Part model, mm, in its own coordinate system. A direction names the side the tool comes from. Round coordinates to 2 decimals unless told otherwise and drop trailing zeros. Loops run counter-clockwise (first coordinate to the right, second up) from the corner with the lowest first, then second, coordinate; pieces in that order, holes last. Notation, with made-up numbers: (5.25, 80) -> (14.25, 80) arc R21 cw to (14.25, 103) -> close; hole circle Ø7 at (69.25, 60.5). An arc over 180 degrees is marked (long way). Answer as a JSON object with one key per item and string values. Group by question number.
from build123d import *

# Parameters (mm, degrees)
CUT_EXTRUDE1_DEPTH      = 127.059509756
CUT_EXTRUDE1_DEPTH_BACK = 127.059509756
SKETCH3_OUTSIDE_W       = 84.264
SKETCH3_OUTSIDE_H       = 84.264
SKETCH3_OUTSIDE_R       = 19
CHAMFER1_SIZE           = 1
CUT_EXTRUDE2_DEPTH      = 148.885090526
CUT_EXTRUDE2_DEPTH_BACK = 148.885090526
SKETCH6_R               = 5
CHAMFER3_SIZE           = 2


with BuildPart() as part:
    # Sketch2 → Revolve1 (revolve)
    with BuildSketch(Plane.XY, mode=Mode.PRIVATE) as revolve1_sk:
        Polygon((0, 0), (145, 0), (145, 15), (39, 15), (39, 25), (24, 25), (24, 15.2), (0, 15.2), align=None)
    revolve(revolve1_sk.sketch.rotate(Axis((0, 0, 0), (1, 0, 0)), 90), axis=Axis((0, 0, 0), (1, 0, 0)))

    # Sketch3 outside → Cut-Extrude1 (cut, two sides: drawn at the far end of the back side and taken through both)
    with BuildSketch(Plane.ZY.offset(-24).offset(-CUT_EXTRUDE1_DEPTH_BACK)):
        Rectangle(SKETCH3_OUTSIDE_W, SKETCH3_OUTSIDE_H)
        with Locations((0, 3)):
            Circle(SKETCH3_OUTSIDE_R, mode=Mode.SUBTRACT)
    extrude(amount=CUT_EXTRUDE1_DEPTH + CUT_EXTRUDE1_DEPTH_BACK, mode=Mode.SUBTRACT)

    # Sketch4 → Cut-Revolve1 (revolve, cut)
    with BuildSketch(Plane.XY, mode=Mode.PRIVATE) as cut_revolve1_sk:
        with BuildLine():
            Line((-1.227130196, 15), (21, 15))
            Line((21, 15), (22.5, 14.133974596))
            ThreePointArc((22.5, 14.133974596), (23.5, 14.133974596), (24, 15))
            Line((24, 15), (24, 19.086801748))
            Line((24, 19.086801748), (-1.227130196, 19.086801748))
            Line((-1.227130196, 19.086801748), (-1.227130196, 15))
        make_face()
        with BuildLine():
            Line((147.328192088, 15), (42, 15))
            Line((42, 15), (40.5, 14.133974596))
            ThreePointArc((40.5, 14.133974596), (39.5, 14.133974596), (39, 15))
            Line((39, 15), (39, 21.506103324))
            Line((39, 21.506103324), (147.328192088, 21.506103324))
            Line((147.328192088, 21.506103324), (147.328192088, 15))
        make_face()
    revolve(cut_revolve1_sk.sketch.rotate(Axis((0, 0, 0), (1, 0, 0)), 90), axis=Axis((0, 0, 0), (1, 0, 0)), mode=Mode.SUBTRACT)

    # Chamfer1
    chamfer1_edges = [part.edges().sort_by_distance(p)[0] for p in [
        (39, 3, -19),
        (24, 3, -19),
    ]]
    chamfer(chamfer1_edges, length=CHAMFER1_SIZE - 0.0001)  # a hair under: the kernel refuses the full size

    # Sketch6 → Cut-Extrude2 (cut, two sides: drawn at the far end of the back side and taken through both)
    with BuildSketch(Plane.ZY.offset(-CUT_EXTRUDE2_DEPTH_BACK)):
        Circle(SKETCH6_R)
    extrude(amount=CUT_EXTRUDE2_DEPTH + CUT_EXTRUDE2_DEPTH_BACK, mode=Mode.SUBTRACT)

    # Chamfer3
    chamfer3_edges = [part.edges().sort_by_distance(p)[0] for p in [
        (0, 0, -15),
        (145, 0, -5),
        (0, 0, -5),
        (145, 0, -15),
    ]]
    chamfer(chamfer3_edges, length=CHAMFER3_SIZE)


solid = part.part
Item 1: Drill centre lines: line 1 (Y direction, x = 108.5, z = 0); line 2 (Y direction, x = 37, z = 0); line 3 (X direction, y = -0.5, z = 17.5). Where is each one in solid material? Low to high.
Item 2: Which spindle directions (+Z, -Z, +X, -X, +Y, -Y) get a long thin tool onto all of the face, cutting with end or side? Do faces 1 (the face through (73.49, -4.88, -1.08)), 2 (the face through (91.79, -12.65, 8.06)), 3 (the face through (11.63, -12.65, 8.06)). Say none if no direction does.
Item 3: Band-saw the part on A-A, the plane x = 19.5. List the corners of the cut face in (y, z).
Item 4: Drop flat-ended pins along their axis: pin 1 Ø13 at (y, z) = (0, 0) entering from -X; pin 2 Ø12 at (x, z) = (123.5, 12) entering from -Y; pin 3 Ø8 at (x, z) = (36.5, 4.5) entering from +Y. Give the stop position or say it passes through.
Entries:
{
 "1": {"line 1": "-15 to -5, 5 to 15", "line 2": "-16 to -5, 5 to 22", "line 3": "24 to 39"},
 "2": {"face 1": "+X, -X", "face 2": "+X", "face 3": "-X"},
 "3": {"outline": "circle Ø30 at (0, 0); hole circle Ø10 at (0, 0)"},
 "4": {"pin 1": "x = 0.5", "pin 2": "y = -13.75", "pin 3": "y = 21.99"}
}
